```python
from build123d import *

# Parameters (mm, degrees)
BOSS_EXTRUDE1_DEPTH = 51.6
CUT_EXTRUDE1_DEPTH  = 10
FILLET3_R           = 4
SKETCH4_W           = 5
SKETCH4_H           = 21.6
BOSS_EXTRUDE2_DEPTH = 2.5
SKETCH5_W           = 21.6
SKETCH5_H           = 1.5
BOSS_EXTRUDE3_DEPTH = 2
SKETCH6_R           = 1.25
CUT_EXTRUDE2_DEPTH  = 2


with BuildPart() as part:
    # Sketch1 → Boss-Extrude1 (new body)
    with BuildSketch(Plane.XY):
        Polygon((-22.497058746, 23.5), (-22.497058746, 22.498632165), (42.604598318, 22.498632165), (46.5, 22.498632165), (46.502941254, 18.5), (46.502941254, 1.893175959), (47.502941254, 1.893175959), (47.502941254, 18.5), (47.502941254, 23.5), (42.5, 23.5), align=None)
    extrude(amount=BOSS_EXTRUDE1_DEPTH)

    # Sketch3 → Cut-Extrude1 (cut)
    with BuildSketch(Plane(origin=(47.502941254, 0, 0), x_dir=(0, 0, -1), z_dir=(1, 0, 0))):
        Polygon((-51.6, 21.5), (-51.6, 1.893175959), (-50.6, 1.893175959), align=None)
        Polygon((0, 21.5), (-1, 1.893175959), (0, 1.893175959), align=None)
    extrude(amount=-CUT_EXTRUDE1_DEPTH, mode=Mode.SUBTRACT)

    # Fillet3
    fillet3_edges = [part.edges().sort_by_distance(p)[0] for p in [
        (46.5, 22.498632165, 25.8),
    ]]
    fillet(fillet3_edges, radius=FILLET3_R)
    fillet3_2_edges = [part.edges().sort_by_distance(p)[0] for p in [
        (47.502941254, 23.5, 25.8),
    ]]
    fillet(fillet3_2_edges, radius=FILLET3_R)

    # Sketch4 → Boss-Extrude2 (add)
    with BuildSketch(Plane.XZ.offset(-22.498632165)):
        with Locations((-19.997058746, 25.8)):
            Rectangle(SKETCH4_W, SKETCH4_H)
    extrude(amount=BOSS_EXTRUDE2_DEPTH)

    # Sketch5 → Boss-Extrude3 (add)
    with BuildSketch(Plane.ZY.offset(22.497058746)):
        with Locations((25.8, 20.748632165)):
            Rectangle(SKETCH5_W, SKETCH5_H)
    extrude(amount=BOSS_EXTRUDE3_DEPTH)

    # Sketch6 → Cut-Extrude2 (cut)
    with BuildSketch(Plane(origin=(47.502941254, 0, 0), x_dir=(0, 0, -1), z_dir=(1, 0, 0))):
        with Locations((-40.048997349, 10.696587979)):
            Circle(SKETCH6_R)
        with Locations((-11.551002651, 10.696587979)):
            Circle(SKETCH6_R)
    extrude(amount=-CUT_EXTRUDE2_DEPTH, mode=Mode.SUBTRACT)


solid = part.part
```
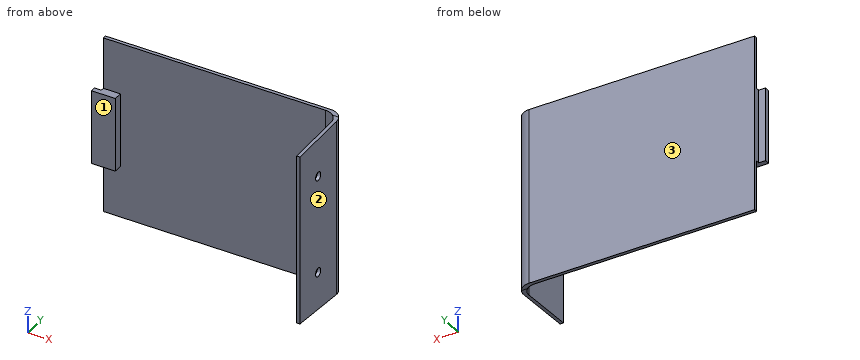
Can you work these out from the model? Positions are in its coordinate system, mm. Face numbers are marked on the shaded views. Give positions to 0.01 mm unless a question says otherwise; leave off trailing zeros. Loops run counter-clockwise (first coordinate to the right, second up) from the corner with the lowest first, then second, coordinate; pieces in that order, holes last. Notation, with made-up numbers: M 47.5,25 L 93.5,25 A25 cw 93.5,51 Z; hole C 28,16 d8. An arc over 180 degrees is marked long. Use CSV: the item, a comma, the result in double quotes. Start each with the question number.
1. If I drill on L1, parallel to X at y = 7.25, z = 22; L2, parallel to Y at x = 29, z = 10.5; L3, parallel to X at y = 22, z = 11, over which ranges is the centre line in solid material (lowest first)?
2. Imagine slicing it at D-D, the plane y = 15.5. Write out the boundary of the cut face in (x, z), plus the area to 3 significant figures.
3. Imagine slicing it at C-C, the plane x = -8. Write out the boundary of the cut face in (y, z).
4. If we mould it in two halves opening along Y, with no side actions, what happens to the marked faces 1, 2 and 3? For each: released by +Y, released by -Y, zero draft, split by the parting line, or undercut.
5. For P1, Ø0.6, axis at y = 22.5, z = 38.5, coming from the -X side; P2, Ø3.5, axis at x = -20.5, z = 27.5, coming from the -Y side; P3, Ø12, axis at y = 9.5, z = 22, coming from the -X side; P4, Ø1.5, axis at y = 10.7, z = 11.55, coming from the +X side, each with a flat end and sliding along its axis, tell me the tip position at first contact or that it passes through.
Response values:
1,L1,"46.5 to 47.5"
1,L2,"22.5 to 23.5"
1,L3,"44.44 to 46.63"
2,outline,"M 46.5,0.31 L 47.5,0.31 L 47.5,51.29 L 46.5,51.29 Z"
2,area,"51.0 mm^2"
3,outline,"M 22.5,0 L 23.5,0 L 23.5,51.6 L 22.5,51.6 Z"
4,face 1,"released by -Y"
4,face 2,"zero draft"
4,face 3,"released by +Y"
5,P1,"x = -22.5"
5,P2,"y = 20"
5,P3,"x = 46.5"
5,P4,"through"
